Can you work these out from the model? Positions are in its coordinate system, mm. A direction names the side the tool comes from. Give positions to 0.01 mm unless a question says otherwise; leave off trailing zeros. Order: outer loops, then holes, each group sorted by start corner. A loop starts at its lowest first (then second) coordinate and runs counter-clockwise, first axis right, second up. Notation, with made-up numbers: M -24,38 L -5,38 A16 ccw -5,63 Z; hole C 89.5,-23 d7. An arc over 180 degrees is marked long. Write each question's results on one line, items separated by ' | '.
from build123d import *

# Parameters (mm, degrees)
F1_DEPTH = 38.1
F2_W     = 69.85
F2_H     = 69.85
F3_DEPTH = 127
F5_DEPTH = 76.2
F7_DEPTH = 5.588
F8_W     = 5.08
F8_H     = 3.175
F9_DEPTH = 76.2


with BuildPart() as f1:
    # F0 (on Right) → F1 (new body, symmetric)
    with BuildSketch(Plane.YZ):
        Polygon((-63.5, 32.0970378816), (-101.6, -44.1029621184), (101.6, -44.1029621184), (63.5, 32.0970378816), align=None)
    extrude(amount=F1_DEPTH, both=True)

    # F2 (on Front) → F3 (cut, symmetric)
    with BuildSketch(Plane.XZ):
        with Locations((0, -6.0029621184)):
            Rectangle(F2_W, F2_H)
    extrude(amount=F3_DEPTH, both=True, mode=Mode.SUBTRACT)

    # F4 (on face) → F5 (cut)
    with BuildSketch(Plane.YZ.offset(38.1)):
        Polygon((-72.39, 2.9578125559), (-93.3803873372, -39.0229621184), (-72.39, -39.0229621184), align=None)
        Polygon((-66.04, 18.0367817605), (-66.04, -39.0229621184), (-8.9802561211, -39.0229621184), align=None)
        Polygon((-3.175, 27.0170378816), (-64.008, 27.0170378816), (-64.008, 24.9850378816), (-3.175, -35.8479621184), align=None)
        Polygon((64.008, 27.0170378816), (3.175, 27.0170378816), (3.175, -35.8479621184), (64.008, 24.9850378816), align=None)
        Polygon((66.04, 18.5374412686), (8.0518, -39.0229621184), (66.04, -39.0229621184), align=None)
        Polygon((72.39, -39.0229621184), (93.3803873372, -39.0229621184), (72.39, 2.9578125559), align=None)
    extrude(amount=-F5_DEPTH, mode=Mode.SUBTRACT)

    # F6 (on face) → F7 (cut)
    with BuildSketch(Plane.XY.offset(32.0970378816)):
        Polygon((-34.925, 51.435), (-34.925, -51.435), (-2.778125, 0), align=None)
        Polygon((0, 4.445), (34.925, 60.325), (-34.925, 60.325), align=None)
        Polygon((2.778125, 0), (34.925, -51.435), (34.925, 51.435), align=None)
        Polygon((-34.925, -60.325), (34.925, -60.325), (0, -4.445), align=None)
    extrude(amount=-F7_DEPTH, mode=Mode.SUBTRACT)

    # F8 (on face) → F9 (join)
    with BuildSketch(Plane.YZ.offset(38.1)):
        with Locations((-99.06, -42.5154621184)):
            Rectangle(F8_W, F8_H)
        with Locations((99.06, -42.5154621184)):
            Rectangle(F8_W, F8_H)
    extrude(amount=-F9_DEPTH)


solid = f1.part
(1) We'd pull the mould along X, two halves only. Please class faces 5 (the face through (18.63, -25.36, 30.53)), 6 (the face through (-36.49, 83.032, -18.326)): +X half, -X half, draft (parallel to the pull), parting line (faces both ways), or undercut.
Data:
face 5: undercut | face 6: draft
(2) Imagine slicing it at C-C, the plane y = -57.5. Write out the boundary of the cut face in (x, z) (3 decimals), plus the area to 3 significant figures.
Data:
outline: M -38.1,-44.103 L 38.1,-44.103 L 38.1,-39.023 L 34.925,-39.023 L 34.925,-40.928 L -34.925,-40.928 L -34.925,-39.023 L -38.1,-39.023 Z; M -38.1,9.497 L -34.925,9.497 L -34.925,18.477 L -38.1,18.477 Z; M -38.1,27.017 L -34.925,27.017 L -34.925,28.922 L -33.159,28.922 L -33.159,32.097 L -38.1,32.097 Z; M 33.159,28.922 L 34.925,28.922 L 34.925,27.017 L 38.1,27.017 L 38.1,32.097 L 33.159,32.097 Z; M 34.925,9.497 L 38.1,9.497 L 38.1,18.477 L 34.925,18.477 Z | area: 355 mm2
(3) Imagine slicing it at B-B, the plane x = 5.5. Write out the boundary of the cut face in (y, z) (1 decimal).
Data:
outline: M -101.6,-44.1 L 101.6,-44.1 L 101.6,-40.9 L -101.6,-40.9 Z; M -65.1,28.9 L -60.3,28.9 L -60.3,32.1 L -63.5,32.1 Z; M -13.2,28.9 L -4.4,28.9 L -4.4,32.1 L -13.2,32.1 Z; M 4.4,28.9 L 13.2,28.9 L 13.2,32.1 L 4.4,32.1 Z; M 60.3,28.9 L 65.1,28.9 L 63.5,32.1 L 60.3,32.1 Z
(4) Imagine slicing it at A-A, the plane y = -12. Count the separate pieces of the cut face and the enclosed holes in it, plus the area to 3 significant figures.
Data:
separate pieces: 7 | enclosed holes: 0 | area: 379 mm2
(5) For faces 1 (the face through (36.535, 33.166, -5.857)), 2 (the face through (1, -1, -44.103)), 3 (the face through (17.71, -32.78, 30.53)), 4 (the face through (0, 63, 28.922)), which set-ups out of +Z, -Z, +X, -X, +Y, -Y let a thin tool reach every point of the face, with its end or its side?
Data:
face 1: +X, -X | face 2: -Z, +X, -X, +Y, -Y | face 3: +Z | face 4: +Y, -Y
(6) I need wall thicknesses on L1, parallel to X at y = 22, z = -22 (3 decimals); L2, parallel to Z at x = 13, y = -35.5. Which ranges of each line are inside material? Lowest first, please. Write a range as from..to.
Data:
L1: x = -38.1..-34.925, 34.925..38.1 | L2: z = -44.1..-40.93
(7) Will these pins go through, and if not, where does the flat tip stop? P1, Ø1.6, axis at x = 36.5, z = -25, coming from the -Y side; P2, Ø2.5, axis at x = -5.5, z = 30.5, coming from the +Y side; P3, Ø1, axis at x = -37, z = 25.5, coming from the -Y side.
Data:
P1: stops at y = -92.45 | P2: stops at y = 64.92 | P3: stops at y = -67.05
